```python
from build123d import *

# Parameters (mm, degrees)
F0_R     = 21
F1_DEPTH = 5
F2_D     = 2
F2_DEPTH = 10
F8_DEPTH = 25


with BuildPart() as f1:
    # F0 (on Top) → F1 (new body)
    with BuildSketch(Plane.XY):
        Circle(F0_R)
    extrude(amount=F1_DEPTH)

    # F2
    with Locations(Plane(origin=(0, 0, 0), x_dir=(1, 0, 0), z_dir=(0, 0, -1))):
        with Locations((0, 9), (15, 0), (0, -9), (-15, 0)):
            Hole(F2_D / 2, depth=F2_DEPTH)

    # F6: sweep along a path in F3
    with BuildLine(Plane.XY) as f6_path:
        CenterArc((0, 0), 12.5, 0, 360)
    # F5 (on Front) → F6 (sweep)
    with BuildSketch(Plane.XZ):
        with BuildLine():
            Line((-11.9, 0), (-13.1, 0))
            ThreePointArc((-13.1, 0), (-12.5, -0.6), (-11.9, 0))
        make_face()
    sweep(path=f6_path.line)

    # F7 (on face) → F8 (cut)
    with BuildSketch(Plane.XY.offset(5)):
        with BuildLine():
            ThreePointArc((1.788854, -1.1), (2.020717, -0.571579), (2.1, 0))
            ThreePointArc((2.1, 0), (2.020717, 0.571579), (1.788854, 1.1))
            Line((1.788854, 1.1), (-1.788854, 1.1))
            ThreePointArc((-1.788854, 1.1), (-2.1, 0), (-1.788854, -1.1))
            Line((-1.788854, -1.1), (1.788854, -1.1))
        make_face()
        with BuildLine():
            ThreePointArc((-1.788854, -1.1), (0, -2.1), (1.788854, -1.1))
            Line((1.788854, -1.1), (-1.788854, -1.1))
        make_face()
        with BuildLine():
            Line((-1.788854, 1.1), (1.788854, 1.1))
            ThreePointArc((1.788854, 1.1), (0, 2.1), (-1.788854, 1.1))
        make_face()
    extrude(amount=-F8_DEPTH, mode=Mode.SUBTRACT)

    # F11: sweep along a path in F9
    with BuildLine(Plane.XY) as f11_path:
        CenterArc((0, 0), 17.5, 0, 360)
    # F10 (on Front) → F11 (sweep)
    with BuildSketch(Plane.XZ):
        with BuildLine():
            Line((18.1, 0), (16.9, 0))
            ThreePointArc((16.9, 0), (17.5, -0.6), (18.1, 0))
        make_face()
    sweep(path=f11_path.line)


solid = f1.part
```
Here's how the part is built. I have some questions about the finished solid (model axes, mm). A direction names the side the tool comes from. Round coordinates to 2 decimals unless told otherwise and drop trailing zeros. Loops run counter-clockwise (first coordinate to the right, second up) from the corner with the lowest first, then second, coordinate; pieces in that order, holes last. Notation, with made-up numbers: (-14.5, 50) -> (4.5, 50) arc R20 cw to (4.5, 60) -> close; hole circle Ø2 at (30, -23.5). An arc over 180 degrees is marked (long way). Answer as CSV lines item,"result". Start each with the question number.
1. I'm going to push flat-ended pins straight in: P1, Ø1.6, axis at x = -15, y = 0, coming from the +Z side; P2, Ø1, axis at y = -10, z = 0, coming from the +X side; P3, Ø3, axis at y = -9, z = 2, coming from the +X side; P4, Ø2, axis at x = 12.5, z = 3, coming from the -Y side. Where does each tip first touch, or does it pass through?
2. I need wall thicknesses on probe 1 along Z at (x, y) = (6.5, -15); probe 2 along Y at (x, z) = (-15, 1.35); probe 3 along Y at (x, z) = (14.5, 3.25). Which ranges of each line are inside material? Lowest first, please. Write a range as from..to.
3. For faces 1 (the face through (-13, 4, 0)), 2 (the face through (-16, 0, 3)), which set-ups out of +Z, -Z, +X, -X, +Y, -Y let a thin tool reach every point of the face, with its end or its side?
4. If we mould it in two halves opening along Y, with no side actions, what happens to faces 3 (the face through (20.03, 6.31, 2.46)), 4 (the face through (4, 0, 5)), 5 (the face through (-0.2, -2.5, 0)), 6 (the face through (0, -10, 3))? For each: pulls with the +Y half, pulls with the -Y half, needs draft (parallel to the pull), parting line crosses it, or undercut.
5. Imagine slicing it at A-A on z = 4.05. Write out the boundary of the cut face in (x, y), plus the area to 3 significant figures.
Solution:
1,P1,"through"
1,P2,"x = 18.73"
1,P3,"x = 19.62"
1,P4,"y = -17.57"
2,probe 1,"0..5"
2,probe 2,"-14.7..-1, 1..14.7"
2,probe 3,"-15.19..-0.87, 0.87..15.19"
3,face 1,"-Z"
3,face 2,"+Z, -Z"
4,face 3,"parting line crosses it"
4,face 4,"needs draft"
4,face 5,"undercut"
4,face 6,"undercut"
5,outline,"circle Ø42 at (0, 0); hole circle Ø2 at (-15, 0); hole (-1.79, -1.1) arc R2.1 ccw to (1.79, -1.1) arc R2.1 ccw to (1.79, 1.1) arc R2.1 ccw to (-1.79, 1.1) arc R2.1 ccw to start; hole circle Ø2 at (0, -9); hole circle Ø2 at (0, 9); hole circle Ø2 at (15, 0)"
5,area,"1,360 mm²"
